Answer from the drawing. Dimensions are ordinates in mm from the lowest x, y and z of the part. Round coordinates to 2 decimals unless told otherwise and drop trailing zeros. Loops run counter-clockwise (first coordinate to the right, second up) from the corner with the lowest first, then second, coordinate; pieces in that order, holes last.
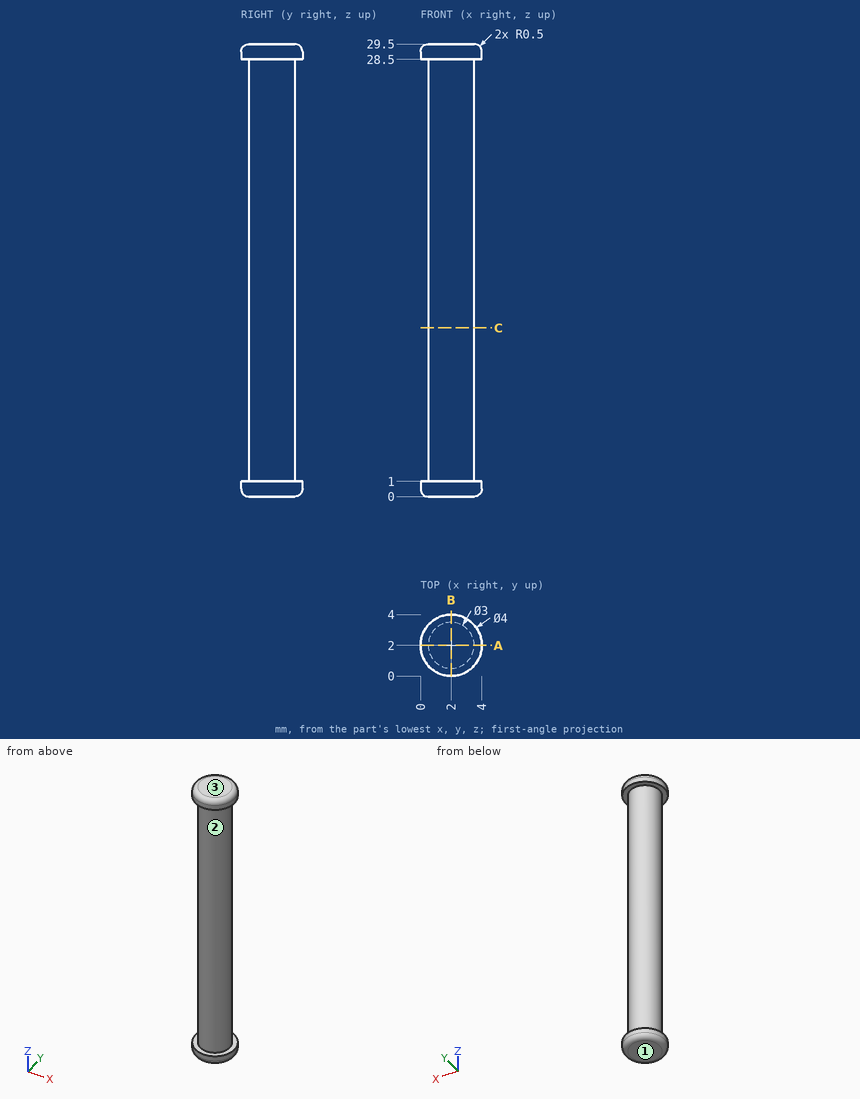
Item 1: Determine the mould class of the marked faces 1, 2 and 3 for opening direction Z: pulls with the +Z half, pulls with the -Z half, needs draft (parallel to the pull), parting line crosses it, or undercut.
Item 2: Section A-A, the plane y = 2 is taken. Give the vertices of the cut face in (x, z), plus the area to 3 significant figures.
Item 3: Section C-C, the plane z = 11 is taken. Give the vertices of the cut face in (x, y).
Item 4: Straight lines are drawn through the part: line 1 (Z direction, x = 1.25, y = 0.55); line 2 (Z direction, x = 0.2, y = 1.6); line 3 (X direction, y = 2.1, z = 6.5). For each, find the intervals that lie inside material, in ascending order.
Item 5: This flat-tipped pin is pushed along its axis until it touches: P1, Ø1, axis at y = 2, z = 14, coming from the -X side. Where does it stop, or does it pass through?
Answer below:
1. face 1: pulls with the -Z half
1. face 2: undercut
1. face 3: pulls with the +Z half
2. outline: (0, 0.5) arc R0.5 ccw to (0.5, 0) - (3.5, 0) arc R0.5 ccw to (4, 0.5) - (4, 1) - (3.5, 1) - (3.5, 28.5) - (4, 28.5) - (4, 29) arc R0.5 ccw to (3.5, 29.5) - (0.5, 29.5) arc R0.5 ccw to (0, 29) - (0, 28.5) - (0.5, 28.5) - (0.5, 1) - (0, 1) - close
2. area: 90.3 mm2
3. outline: circle Ø3 at (2, 2)
4. line 1: z = 0.02 to 1, 28.5 to 29.48
4. line 2: z = 0.14 to 1, 28.5 to 29.36
4. line 3: x = 0.5 to 3.5
5. P1: stops at x = 0.5
